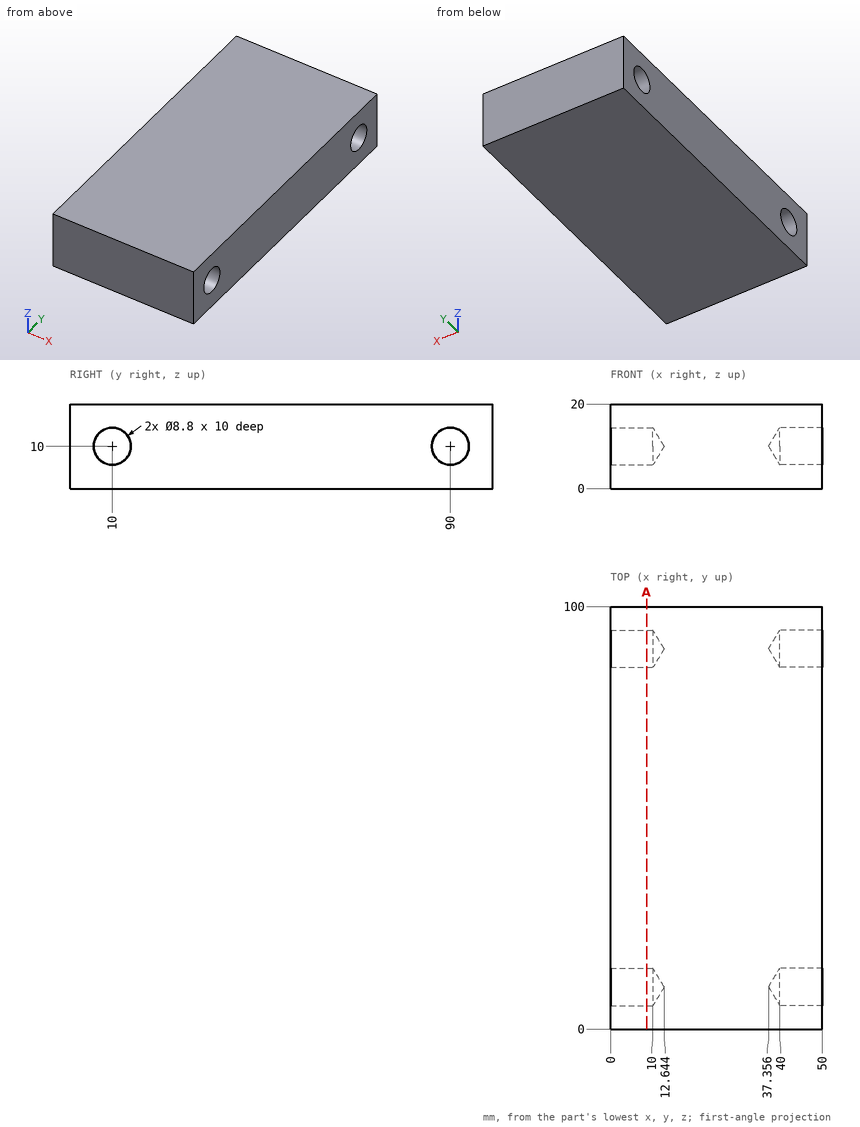
Source: three-view drawing plus pictorial views. Frame: mm from the lowest corner of the part. Round coordinates to 2 decimals unless told otherwise and drop trailing zeros. Order: outer loops, then holes, each group sorted by start corner. A loop starts at its lowest first (then second) coordinate and runs counter-clockwise, first axis right, second up. Notation, with made-up numbers: (62, -7) -> (76, -7) arc R18 cw to (76, 20) -> close; hole circle Ø9 at (27.25, 67). An arc over 180 degrees is marked (long way). Use one line per item in the form item = value.
(1) Ray query, probe 1 along Y at (x, z) = (7.75, 10); probe 2 along Y at (x, z) = (4, 12.5); probe 3 along Z at (x, y) = (6.25, 10). Return the intervals inside material, ascending. Write a range as [from, to].
Results list:
probe_1 = [0, 5.6], [14.4, 85.6], [94.4, 100]
probe_2 = [0, 6.38], [13.62, 86.38], [93.62, 100]
probe_3 = [0, 5.6], [14.4, 20]
(2) First-contact query: pin 1 Ø8 at (y, z) = (10, 10) entering from -X; pin 2 Ø5.5 at (y, z) = (90, 10) entering from -X. Flat tips, straight axial feed; report the tip coordinate or a pass-through.
Results list:
pin_1 = 10.24
pin_2 = 10.99
(3) Section A-A on x = 8.5. Return loops of the section in (y, z), and give its area (3 significant figures).
Results list:
outline = (0, 0) -> (100, 0) -> (100, 20) -> (0, 20) -> close; hole circle Ø8.8 at (10, 10); hole circle Ø8.8 at (90, 10)
area = 1,880 mm^2
